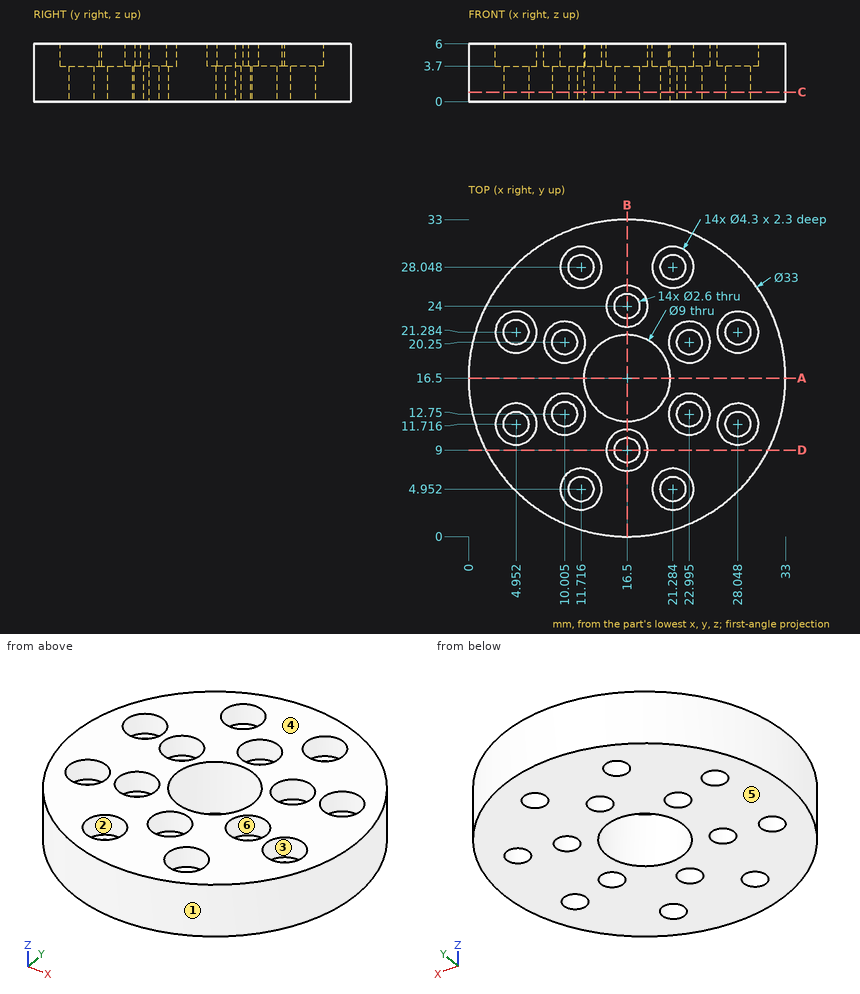
Could you check a few things on this drawing? It's one solid part, dimensions in mm from its lowest x, y, z. A direction names the side the tool comes from. Coordinates: 2 decimals unless noted, no trailing zeros. Loops run counter-clockwise (first coordinate to the right, second up) from the corner with the lowest first, then second, coordinate; pieces in that order, holes last. Notation, with made-up numbers: (25.25, 62) - (48.25, 62) arc R11 ccw to (48.25, 70) - close; hole circle Ø7 at (8.5, 44.5). An arc over 180 degrees is marked (long way). Answer as a JSON object with one key per item and string values. Group by question number.
Item 1: If we section it at B-B (x = 16.5): List the corners of the cut face in (y, z) for me.
Item 2: If we section it at D-D (y = 9): List the corners of the cut face in (x, z) for me.
Item 3: If we mould it in two halves opening along Y, with no side actions, what happens to the marked faces 1, 2, 3 and 4? For each: released by +Y, released by -Y, zero draft, split by the parting line, or undercut.
Item 4: On a 3-axis mill with a long thin cutter (end or side, diameter ignored), from which of +Z, -Z, +X, -X, +Y, -Y can I reach the whole of each face in a straight line? I mean the marked faces 5 and 6. Say none if no direction works.
Item 5: If we section it at A-A (y = 16.5): List the corners of the cut face in (x, z) for me, plus the area to 3 significant figures.
Item 6: For pin 1 (1.5 mm diameter, centred on x = 28.5, y = 18.5, fed in from -Z); pin 2 (2 mm diameter, centred on y = 26.5, z = 1.5, fed in from +X); pin 3 (3 mm diameter, centred on x = 20.5, z = 1, fed in from -Y); pin 4 (3.5 mm diameter, centred on x = 21.28, y = 4.95, fed in from +Z), each with a flat end and sliding along its axis, tell me the tip position at first contact or that it passes through.
Item 7: If we section it at C-C (z = 1): State how many separate pieces and enclosed holes the cut face has.
Item 8: If I drill on L1, parallel to Y at x = 11.5, z = 5.5 (1 decimal); L2, parallel to X at y = 29, z = 1.6 (1 decimal); L3, parallel to X at y = 5.5, z = 3.4 (1 decimal), over which ranges is the centre line in solid material (lowest first)? Write a range as from..to.
Returned:
{
 "1": {"outline": "(0, 0) - (7.7, 0) - (7.7, 3.7) - (6.85, 3.7) - (6.85, 6) - (0, 6) - close; (10.3, 0) - (12, 0) - (12, 6) - (11.15, 6) - (11.15, 3.7) - (10.3, 3.7) - close; (21, 0) - (22.7, 0) - (22.7, 3.7) - (21.85, 3.7) - (21.85, 6) - (21, 6) - close; (25.3, 0) - (33, 0) - (33, 6) - (26.15, 6) - (26.15, 3.7) - (25.3, 3.7) - close"},
 "2": {"outline": "(1.8, 0) - (15.2, 0) - (15.2, 3.7) - (14.35, 3.7) - (14.35, 6) - (1.8, 6) - close; (17.8, 0) - (31.2, 0) - (31.2, 6) - (18.65, 6) - (18.65, 3.7) - (17.8, 3.7) - close"},
 "3": {"face 1": "split by the parting line", "face 2": "undercut", "face 3": "undercut", "face 4": "zero draft"},
 "4": {"face 5": "-Z, +X, -X, +Y, -Y", "face 6": "+Z"},
 "5": {"outline": "(0, 0) - (12, 0) - (12, 6) - (0, 6) - close; (21, 0) - (33, 0) - (33, 6) - (21, 6) - close", "area": "144 mm²"},
 "6": {"pin 1": "stops at z = 0", "pin 2": "stops at x = 30.33", "pin 3": "stops at y = 0.19", "pin 4": "stops at z = 3.7"},
 "7": {"separate pieces": "1", "enclosed holes": "15"},
 "8": {"L1": "y = 0.8..2.8, 7.1..11.2, 14.3..18.7, 21.8..25.9, 30.2..32.2", "L2": "x = 5.7..10.8, 12.6..20.4, 22.2..27.3", "L3": "x = 4.2..10.5, 12.9..20.1, 22.5..28.8"}
}
